```python
from build123d import *

# Parameters (mm, degrees)
CHAMFER2_SIZE      = 1.5875
SKETCH3_R          = 7.1501
CUT_EXTRUDE1_DEPTH = 165.675089552
CIRPATTERN1_COUNT  = 5
FILLET1_R          = 0.762
CHAMFER3_SIZE      = 3.175
CHAMFER3_SIZE2     = 1.5875
SKETCH4_R          = 7.1501
CUT_EXTRUDE2_DEPTH = 165.675089552
SKETCH5_R          = 7.1501
CUT_EXTRUDE3_DEPTH = 165.675089552
CIRPATTERN2_COUNT  = 36
SKETCH8_W          = 12.7
SKETCH8_H          = 15.875
CUT_EXTRUDE4_DEPTH = 172.890277093


with BuildPart() as part:
    # Sketch1 → Revolve1 (revolve)
    with BuildSketch(Plane.XY, mode=Mode.PRIVATE) as revolve1_sk:
        with BuildLine():
            Line((0, 65.0875), (0, 70.0151))
            Line((0, 70.0151), (35.1028, 70.0151))
            Line((35.1028, 70.0151), (35.1028, 113.7666))
            Line((35.1028, 113.7666), (60.5028, 113.7666))
            Line((60.5028, 113.7666), (60.5028, 41.275))
            Line((60.5028, 41.275), (37.1856, 41.275))
            Line((37.1856, 41.275), (37.1856, 54.851738008))
            ThreePointArc((37.1856, 54.851738008), (35.183653306, 59.99973539), (30.22972676, 62.442741607))
            Line((30.22972676, 62.442741607), (0, 65.0875))
        make_face()
    revolve(revolve1_sk.sketch.rotate(Axis((0, 0, 0), (1, 0, 0)), 90), axis=Axis((0, 0, 0), (1, 0, 0)))

    # Chamfer2
    chamfer2_edges = [part.edges().sort_by_distance(p)[0] for p in [
        (60.5028, 0, -41.275),
    ]]
    chamfer(chamfer2_edges, length=CHAMFER2_SIZE)

    # Sketch3 → Cut-Extrude1 (cut, through all)
    with BuildSketch(Plane.ZY.offset(-35.1028)):
        with Locations((0, 98.425)):
            Circle(SKETCH3_R)
    cut_extrude1 = extrude(amount=-CUT_EXTRUDE1_DEPTH, mode=Mode.SUBTRACT)

    # CirPattern1: Cut-Extrude1 ×5 about axis
    cirpattern1_axis = Axis((0, 0, 0), (1, 0, 0))
    for i in range(1, CIRPATTERN1_COUNT):
        add(cut_extrude1.rotate(cirpattern1_axis, i * 360 / CIRPATTERN1_COUNT), mode=Mode.SUBTRACT)

    # Fillet1
    fillet1_edges = [part.edges().sort_by_distance(p)[0] for p in [
        (35.1028, 0, -70.0151),
    ]]
    fillet(fillet1_edges, radius=FILLET1_R)

    # Chamfer3
    chamfer3_edges = [part.edges().sort_by_distance(p)[0] for p in [
        (0, 0, -70.0151),
    ]]
    chamfer3_side = [part.faces().sort_by_distance(p)[0] for p in [
        (17.1704, 0, -70.0151),
    ]]
    chamfer(chamfer3_edges, length=CHAMFER3_SIZE, length2=CHAMFER3_SIZE2, reference=chamfer3_side[0])

    # Sketch4 → Cut-Extrude2 (cut, through all)
    with BuildSketch(Plane.ZY.offset(-35.1028)):
        with Locations((-98.425, 0)):
            Circle(SKETCH4_R)
    cut_extrude2 = extrude(amount=-CUT_EXTRUDE2_DEPTH, mode=Mode.SUBTRACT)

    # Mirror1: Cut-Extrude2 across plane
    add(cut_extrude2.mirror(Plane.XY), mode=Mode.SUBTRACT)

    # Sketch5 → Cut-Extrude3 (cut, through all)
    with BuildSketch(Plane.ZY.offset(-35.1028)):
        with Locations((0, -98.425)):
            Circle(SKETCH5_R)
    cut_extrude3 = extrude(amount=-CUT_EXTRUDE3_DEPTH, mode=Mode.SUBTRACT)

    # CirPattern2: Cut-Extrude3 ×36 about axis, 33 skipped
    cirpattern2_axis = Axis((0, 0, 0), (-1, 0, 0))
    add([cut_extrude3.rotate(cirpattern2_axis, i * 360 / CIRPATTERN2_COUNT) for i in range(1, CIRPATTERN2_COUNT) if i not in (1, 2, 3, 4, 5, 6, 7, 8, 9, 10, 11, 12, 14, 15, 16, 17, 18, 19, 20, 21, 22, 24, 25, 26, 27, 28, 29, 30, 31, 32, 33, 34, 35)], mode=Mode.SUBTRACT)

    # Sketch7 → Cut-Revolve1 (revolve, cut)
    with BuildSketch(Plane.XY, mode=Mode.PRIVATE) as cut_revolve1_sk:
        Polygon((20.8788, 70.0151), (20.8788, 67.1449), (25.6794, 67.1449), (25.6794, 70.0151), (25.6794, 72.174819971), (20.8788, 72.174819971), align=None)
    revolve(cut_revolve1_sk.sketch.rotate(Axis((-34.095628325, 0, 0), (1, 0, 0)), 270), axis=Axis((-34.095628325, 0, 0), (1, 0, 0)), mode=Mode.SUBTRACT)

    # Sketch8 → Cut-Extrude4 (cut, through all)
    with BuildSketch(Plane(origin=(0, 0, 0), x_dir=(1, 0, 0), z_dir=(0, 1, 0))):
        with Locations((6.35, 0)):
            Rectangle(SKETCH8_W, SKETCH8_H)
    extrude(amount=-CUT_EXTRUDE4_DEPTH, mode=Mode.SUBTRACT)


solid = part.part
```
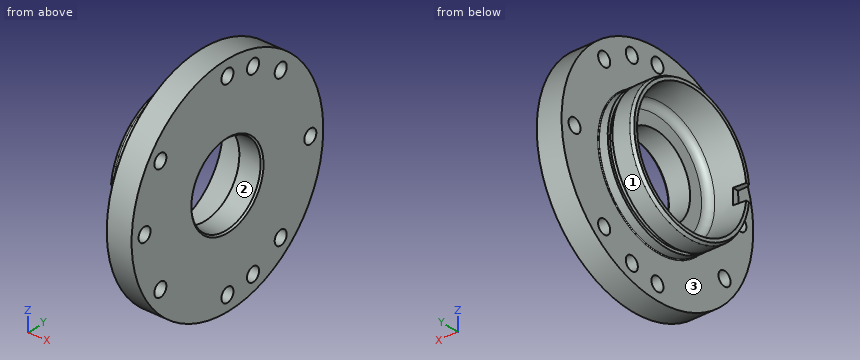
Part model, mm, in its own coordinate system. Face numbers are marked on the shaded views. Round coordinates to 2 decimals unless told otherwise and drop trailing zeros.
Item 1: Two-plate mould, pull along Y, no slides. Class the marked faces 1, 2 and 3: +Y half, -Y half, draft (parallel to the pull), parting line (faces both ways), or undercut.
Results:
face 1: parting line
face 2: undercut
face 3: draft
Item 2: Cut at A-A, the plane y = 0. Count the separate pieces of the cut face and the enclosed holes in it, plus the area to 3 significant figures.
Results:
separate pieces: 4
enclosed holes: 0
area: 3,310 mm2
Item 3: Probe L1, parallel to Y at x = 40.75, z = 0 (3 decimals); L2, parallel to Y at x = 45, z = -95; L3, parallel to Y at x = 40.5, z = -99. List the from-to ranges inside material, lowest first.
Results:
L1: y = -113.767 to -105.575, -91.275 to -41.275, 41.275 to 91.275, 105.575 to 113.767
L2: y = -62.59 to -6.28, 6.28 to 23.4, 37.43 to 62.59
L3: y = -56.05 to -7.13, 7.13 to 25.72, 35.11 to 56.05
Item 4: Drop flat-ended pins along their axis: pin 1 Ø8.5 at (y, z) = (63.27, 75.4) entering from -X (3 decimals); pin 2 Ø12 at (x, z) = (41.5, -46) entering from +Y; pin 3 Ø23 at (y, z) = (63.27, -75.4) entering from +X; pin 4 Ø3 at (x, z) = (43.5, 33) entering from +Y. Give the stop position or say it passes through.
Results:
pin 1: passes through
pin 2: stops at y = 106.5
pin 3: stops at x = 60.5
pin 4: stops at y = 109.32
